from build123d import *
from build123d.topology import SkipClean

# Parameters (mm, degrees)
BOSS_EXTRUDE1_DEPTH           = 3
BOSS_EXTRUDE2_START           = -1.75
SKETCH1_3_R                   = 11
BOSS_EXTRUDE2_DEPTH           = 1.75
SKETCH2_R                     = 1.75
CUT_EXTRUDE1_DEPTH            = 4.75
SKETCH2_3_R                   = 3
CUT_EXTRUDE2_DEPTH            = 3.75
SKETCH1_6_W                   = 11
SKETCH1_6_H                   = 5.31
BOSS_EXTRUDE3_DEPTH           = 6
SKETCH3_R                     = 1.1
CUT_EXTRUDE3_DEPTH            = 9
SKETCH3_3_R                   = 2
SKETCH3_3_R_2                 = 1.1
CUT_EXTRUDE4_DEPTH            = 8
BODY_MOVE_COPY1_START         = -3
BODY_MOVE_COPY1_OUTLINE_R     = 3
BODY_MOVE_COPY1_DEPTH         = 3
BODY_MOVE_COPY1_START_2       = 3
BODY_MOVE_COPY1_2_OUTLINE_W   = 22
BODY_MOVE_COPY1_2_OUTLINE_H   = 5.31
BODY_MOVE_COPY1_2_OUTLINE_R   = 2
BODY_MOVE_COPY1_2_DEPTH       = 3
BODY_MOVE_COPY1_START_3       = 0.75
BODY_MOVE_COPY1_3_OUTLINE_R   = 3
BODY_MOVE_COPY1_3_OUTLINE_R_2 = 1.75
BODY_MOVE_COPY1_3_DEPTH       = 1
BODY_MOVE_COPY1_START_4       = 5
BODY_MOVE_COPY1_4_OUTLINE_R   = 2
BODY_MOVE_COPY1_4_OUTLINE_R_2 = 1.1
BODY_MOVE_COPY1_4_DEPTH       = 1
BODY_MOVE_COPY1_5_DEPTH       = 3
BODY_MOVE_COPY1_START_5       = 1.75
BODY_MOVE_COPY1_6_OUTLINE_R   = 11
BODY_MOVE_COPY1_6_OUTLINE_R_2 = 3
BODY_MOVE_COPY1_6_DEPTH       = 1.25
BODY_MOVE_COPY1_START_6       = -6
BODY_MOVE_COPY1_7_OUTLINE_W   = 22
BODY_MOVE_COPY1_7_OUTLINE_H   = 5.31
BODY_MOVE_COPY1_7_OUTLINE_R   = 1.1
BODY_MOVE_COPY1_7_DEPTH       = 3
BODY_MOVE_COPY1_START_7       = -1.75
BODY_MOVE_COPY1_8_OUTLINE_R   = 3
BODY_MOVE_COPY1_8_OUTLINE_R_2 = 1.75
BODY_MOVE_COPY1_8_DEPTH       = 1


# Read off the part's stored shape, not the designer's step: Body-Move/Copy1
with BuildPart() as part:
    # Sketch1 → Boss-Extrude1 (new body)
    with BuildSketch(Plane.XY):
        with BuildLine():
            Line((-11, 29.175), (-11, -29.175))
            Line((-11, -29.175), (11, -29.175))
            Line((11, -29.175), (11, 29.175))
            ThreePointArc((11, 29.175), (0, 40.175), (-11, 29.175))
        make_face()
        with BuildLine():
            Line((5, -22.865), (-5, -22.865))
            Line((-5, -22.865), (-5, 18.818842411))
            ThreePointArc((-5, 18.818842411), (0, 17.675), (5, 18.818842411))
            Line((5, 18.818842411), (5, -22.865))
        make_face(mode=Mode.SUBTRACT)
    extrude(amount=BOSS_EXTRUDE1_DEPTH)

    # Sketch1<3> → Boss-Extrude2 (add)
    with BuildSketch(Plane.XY.offset(BOSS_EXTRUDE2_START)):
        with Locations((0, 29.175)):
            Circle(SKETCH1_3_R)
    extrude(amount=BOSS_EXTRUDE2_DEPTH)

    # Sketch2 → Cut-Extrude1 (cut)
    with BuildSketch(Plane.XY.offset(3)):
        with Locations((0, 29.175)):
            Circle(SKETCH2_R)
    extrude(amount=-CUT_EXTRUDE1_DEPTH, mode=Mode.SUBTRACT)

    # Sketch2<3> → Cut-Extrude2 (cut)
    with BuildSketch(Plane.XY.offset(3)):
        with Locations((0, 29.175)):
            Circle(SKETCH2_3_R)
    extrude(amount=-CUT_EXTRUDE2_DEPTH, mode=Mode.SUBTRACT)

    # Sketch1<6> → Boss-Extrude3 (add)
    with BuildSketch(Plane.XY):
        with Locations((5.5, -26.52)):
            Rectangle(SKETCH1_6_W, SKETCH1_6_H)
        with Locations((-5.5, -26.52)):
            Rectangle(SKETCH1_6_W, SKETCH1_6_H)
    extrude(amount=-BOSS_EXTRUDE3_DEPTH)

    # Sketch3 → Cut-Extrude3 (cut)
    with BuildSketch(Plane.XY.offset(3)):
        with Locations((-8.5, -26.67999607)):
            Circle(SKETCH3_R)
        with Locations((8.5, -26.67999607)):
            Circle(SKETCH3_R)
    extrude(amount=-CUT_EXTRUDE3_DEPTH, mode=Mode.SUBTRACT)

    # Sketch3<3> → Cut-Extrude4 (cut)
    # profile 1 of 2: a face of its own
    with BuildSketch(Plane.XY.offset(3)):
        with Locations((-8.5, -26.67999607)):
            Circle(SKETCH3_3_R)
        with Locations((-8.5, -26.67999607)):
            Circle(SKETCH3_3_R_2, mode=Mode.SUBTRACT)
    # profile 2 of 2: a face of its own
    with BuildSketch(Plane.XY.offset(3)):
        with Locations((8.5, -26.67999607)):
            Circle(SKETCH3_3_R)
        with Locations((8.5, -26.67999607)):
            Circle(SKETCH3_3_R_2, mode=Mode.SUBTRACT)
    extrude(amount=-CUT_EXTRUDE4_DEPTH, mode=Mode.SUBTRACT)

    # Body-Move/Copy1 outline → Body-Move/Copy1 (add)
    with BuildSketch(Plane.XY.offset(BODY_MOVE_COPY1_START)):
        with BuildLine():
            Line((-11, 29.175), (-11, -23.865))
            Line((-11, -23.865), (11, -23.865))
            Line((11, -23.865), (11, 29.175))
            ThreePointArc((11, 29.175), (0, 40.175), (-11, 29.175))
        make_face()
        with BuildLine():
            Line((-5, -22.865), (-5, 18.818842411))
            ThreePointArc((-5, 18.818842411), (0, 17.675), (5, 18.818842411))
            Line((5, 18.818842411), (5, -22.865))
            Line((5, -22.865), (-5, -22.865))
        make_face(mode=Mode.SUBTRACT)
        with Locations((0, 29.175)):
            Circle(BODY_MOVE_COPY1_OUTLINE_R, mode=Mode.SUBTRACT)
    extrude(amount=BODY_MOVE_COPY1_DEPTH)

    # Body-Move_Copy1 2 outline → Body-Move_Copy1 2 (add)
    with BuildSketch(Plane.XY.offset(BODY_MOVE_COPY1_START_2)):
        with Locations((0, -26.52)):
            Rectangle(BODY_MOVE_COPY1_2_OUTLINE_W, BODY_MOVE_COPY1_2_OUTLINE_H)
        with Locations((-8.5, -26.67999607)):
            Circle(BODY_MOVE_COPY1_2_OUTLINE_R, mode=Mode.SUBTRACT)
        with Locations((8.5, -26.67999607)):
            Circle(BODY_MOVE_COPY1_2_OUTLINE_R, mode=Mode.SUBTRACT)
    extrude(amount=BODY_MOVE_COPY1_2_DEPTH)

    # Body-Move_Copy1 3 outline → Body-Move_Copy1 3 (add)
    with BuildSketch(Plane.XY.offset(BODY_MOVE_COPY1_START_3)):
        with Locations((0, 29.175)):
            Circle(BODY_MOVE_COPY1_3_OUTLINE_R)
        with Locations((0, 29.175)):
            Circle(BODY_MOVE_COPY1_3_OUTLINE_R_2, mode=Mode.SUBTRACT)
    extrude(amount=BODY_MOVE_COPY1_3_DEPTH)

    # Body-Move_Copy1 4 outline → Body-Move_Copy1 4 (add)
    # profile 1 of 2: a face of its own
    with BuildSketch(Plane.XY.offset(BODY_MOVE_COPY1_START_4)):
        with Locations((-8.5, -26.67999607)):
            Circle(BODY_MOVE_COPY1_4_OUTLINE_R)
        with Locations((-8.5, -26.67999607)):
            Circle(BODY_MOVE_COPY1_4_OUTLINE_R_2, mode=Mode.SUBTRACT)
    # profile 2 of 2: a face of its own
    with BuildSketch(Plane.XY.offset(BODY_MOVE_COPY1_START_4)):
        with Locations((8.5, -26.67999607)):
            Circle(BODY_MOVE_COPY1_4_OUTLINE_R)
        with Locations((8.5, -26.67999607)):
            Circle(BODY_MOVE_COPY1_4_OUTLINE_R_2, mode=Mode.SUBTRACT)
    extrude(amount=BODY_MOVE_COPY1_4_DEPTH)

    # Body-Move_Copy1 5 outline → Body-Move_Copy1 5 (cut)
    with SkipClean():  # the faces are left unmerged after this step: merging them gives an invalid solid
        with BuildSketch(Plane.XY):
            with BuildLine():
                Line((-11, 29.175), (-11, -23.865))
                Line((-11, -23.865), (11, -23.865))
                Line((11, -23.865), (11, 29.175))
                ThreePointArc((11, 29.175), (0, 18.175), (-11, 29.175))
            make_face()
            with BuildLine():
                Line((-5, -22.865), (-5, 18.818842411))
                ThreePointArc((-5, 18.818842411), (0, 17.675), (5, 18.818842411))
                Line((5, 18.818842411), (5, -22.865))
                Line((5, -22.865), (-5, -22.865))
            make_face(mode=Mode.SUBTRACT)
        extrude(amount=BODY_MOVE_COPY1_5_DEPTH, mode=Mode.SUBTRACT)

    # Body-Move_Copy1 6 outline → Body-Move_Copy1 6 (cut)
    with BuildSketch(Plane.XY.offset(BODY_MOVE_COPY1_START_5)):
        with Locations((0, 29.175)):
            Circle(BODY_MOVE_COPY1_6_OUTLINE_R)
        with Locations((0, 29.175)):
            Circle(BODY_MOVE_COPY1_6_OUTLINE_R_2, mode=Mode.SUBTRACT)
    extrude(amount=BODY_MOVE_COPY1_6_DEPTH, mode=Mode.SUBTRACT)

    # Body-Move_Copy1 7 outline → Body-Move_Copy1 7 (cut)
    with BuildSketch(Plane.XY.offset(BODY_MOVE_COPY1_START_6)):
        with Locations((0, -26.52)):
            Rectangle(BODY_MOVE_COPY1_7_OUTLINE_W, BODY_MOVE_COPY1_7_OUTLINE_H)
        with Locations((-8.5, -26.67999607)):
            Circle(BODY_MOVE_COPY1_7_OUTLINE_R, mode=Mode.SUBTRACT)
        with Locations((8.5, -26.67999607)):
            Circle(BODY_MOVE_COPY1_7_OUTLINE_R, mode=Mode.SUBTRACT)
    extrude(amount=BODY_MOVE_COPY1_7_DEPTH, mode=Mode.SUBTRACT)

    # Body-Move_Copy1 8 outline → Body-Move_Copy1 8 (cut)
    with SkipClean():  # the faces are left unmerged after this step: merging them gives an invalid solid
        with BuildSketch(Plane.XY.offset(BODY_MOVE_COPY1_START_7)):
            with Locations((0, 29.175)):
                Circle(BODY_MOVE_COPY1_8_OUTLINE_R)
            with Locations((0, 29.175)):
                Circle(BODY_MOVE_COPY1_8_OUTLINE_R_2, mode=Mode.SUBTRACT)
        extrude(amount=BODY_MOVE_COPY1_8_DEPTH, mode=Mode.SUBTRACT)
    add(part.part.scale(1), mode=Mode.REPLACE)  # the faces are merged on a copy


solid = part.part
Design review of the part built by this model. Coordinates are the model's own, in mm. A direction names the side the tool comes from. Coordinates: 2 decimals unless noted, no trailing zeros. Loops run counter-clockwise (first coordinate to the right, second up) from the corner with the lowest first, then second, coordinate; pieces in that order, holes last.
Item 1: Add section C-C (x = 8.5). Write out the cut boundary in (y, z) (3 decimals).
Completed:
outline: (-29.175, -3) - (-28.68, -3) - (-28.68, 5) - (-27.78, 5) - (-27.78, 6) - (-29.175, 6) - close; (-25.58, 5) - (-24.68, 5) - (-24.68, -3) - (36.157, -3) - (36.157, 1.75) - (22.193, 1.75) - (22.193, 0) - (-23.865, 0) - (-23.865, 6) - (-25.58, 6) - close
Item 2: For faces 5 (the flat face through (0, -26, 6)), 6 (the flat face through (5, -2, -2)), 7 (the flat face through (0, -23.865, 3)), 8 (the flat face through (-8, -28, 5)), list the 3-axis set-ups (+Z, -Z, +X, -X, +Y, -Y) from which the entire face can be reached by the end or side of a thin tool; tool diameter is ignored.
Completed:
face 5: +Z, +X, -X, +Y, -Y
face 6: +Z, -Z
face 7: +Z, +X, -X
face 8: -Z
Item 3: Add section D-D (y = 23). Write out the cut boundary in (x, z).
Completed:
outline: (-11, -3) - (11, -3) - (11, 0) - (9.1, 0) - (9.1, 1.75) - (-9.1, 1.75) - (-9.1, 0) - (-11, 0) - close
Item 4: Add section A-A (x = 0). Write out the cut boundary in (y, z) (3 decimals).
Completed:
outline: (-29.175, -3) - (-22.865, -3) - (-22.865, 0) - (-23.865, 0) - (-23.865, 6) - (-29.175, 6) - close; (17.675, -3) - (26.175, -3) - (26.175, 0.75) - (27.425, 0.75) - (27.425, 1.75) - (18.175, 1.75) - (18.175, 0) - (17.675, 0) - close; (30.925, 0.75) - (32.175, 0.75) - (32.175, -3) - (40.175, -3) - (40.175, 1.75) - (30.925, 1.75) - close
Item 5: Add section B-B (y = -17.5). Write out the cut boundary in (x, z), and give its area (3 significant figures).
Completed:
outline: (-11, -3) - (-5, -3) - (-5, 0) - (-11, 0) - close; (5, -3) - (11, -3) - (11, 0) - (5, 0) - close
area: 36.0 mm2
Item 6: Wall thickness on L1, parallel to Y at x = 0, z = -1.5 (3 decimals); L2, parallel to Y at x = 0, z = 0.5 (3 decimals); L3, parallel to X at y = 15.5, z = -0.75: over which ranges is each line inside the solid? List them lowest first.
Completed:
L1: y = -29.175 to -22.865, 17.675 to 26.175, 32.175 to 40.175
L2: y = -29.175 to -23.865, 18.175 to 26.175, 32.175 to 40.175
L3: x = -11 to -5, 5 to 11
Item 7: Draft analysis for pull direction X (two halves, no side actions). For faces 1 (the flat face through (0, -29.175, 1)), 2 (the flat face through (0, -22.865, -2)), 3 (the flat face through (-11, -7, -1)), 4 (the flat face through (11, -7, -1)), state which applies: pulls with the +X half, pulls with the -X half, needs draft (parallel to the pull), parting line crosses it, or undercut.
Completed:
face 1: needs draft
face 2: undercut
face 3: pulls with the -X half
face 4: pulls with the +X half
Item 8: Clearance check with flat-ended pins moving along their axes: pin 1 (5.5 mm diameter, centred on x = 0, y = 29.175, fed in from +Z); pin 2 (5.5 mm diameter, centred on x = 0, y = 29.175, fed in from -Z); pin 3 (0.9 mm diameter, centred on x = 2, z = -2, fed in from +Y); pin 4 (9.5 mm diameter, centred on x = 0, y = 29.175, fed in from -Z). State where each tip first meets the part, or that it passes through.
Completed:
pin 1: stops at z = 1.75
pin 2: stops at z = 0.75
pin 3: stops at y = 40.07
pin 4: stops at z = -3
